Here's the drawing with two shaded views (mm, measured from the low corner). I have some questions. Coordinates: 2 decimals unless noted, no trailing zeros. Order: outer loops, then holes, each group sorted by start corner. A loop starts at its lowest first (then second) coordinate and runs counter-clockwise, first axis right, second up. Notation, with made-up numbers: (85, 74.5) - (93, 74.5) arc R17 cw to (93, 99.5) - close; hole circle Ø6 at (-14.75, 36). An arc over 180 degrees is marked (long way). Answer as a JSON object with one key per item and string values. Group by question number.
(1) Imagine slicing it at B-B, the plane x = 6.75. Write out the boundary of the cut face in (y, z) (1 decimal).
(2) We'd pull the mould along X, two halves only. Please class the marked faces 1, 2 and 3: pulls with the +X half, pulls with the -X half, needs draft (parallel to the pull), parting line crosses it, or undercut.
(3) Will this pin go through, and if not, where does the flat tip stop? P1, Ø1, axis at x = 3, z = 2, coming from the +Y side.
(4) Imagine slicing it at C-C, the plane z = 1.7. Write out the boundary of the cut face in (x, y) (1 decimal), and give its area (3 significant figures).
(5) Please list where these lines run through material, in increasing order: probe 1 along X at (y, z) = (8, 2.3) (1 decimal); probe 2 along Y at (x, z) = (6.5, 1.6) (1 decimal); probe 3 along Y at (x, z) = (5.75, 1.15) (1 decimal).
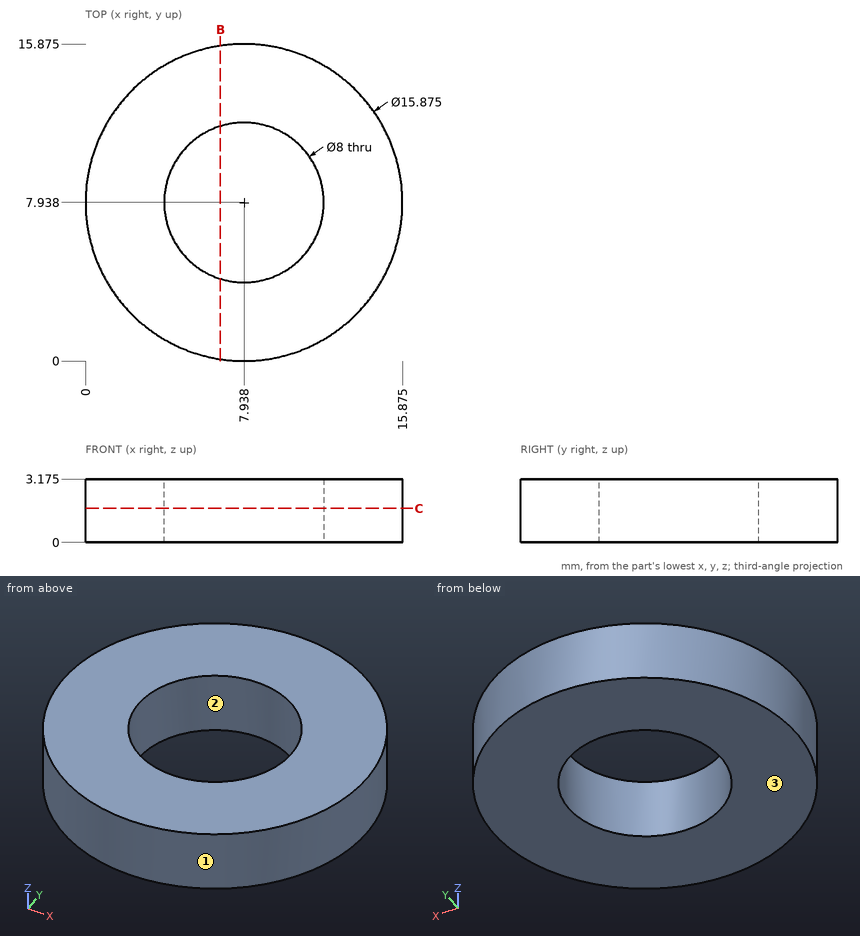
Result set:
{
 "1": {"outline": "(0.1, 0) - (4.1, 0) - (4.1, 3.2) - (0.1, 3.2) - close; (11.8, 0) - (15.8, 0) - (15.8, 3.2) - (11.8, 3.2) - close"},
 "2": {"face 1": "parting line crosses it", "face 2": "undercut", "face 3": "needs draft"},
 "3": {"P1": "stops at y = 14.52"},
 "4": {"outline": "circle Ø15.9 at (7.9, 7.9); hole circle Ø8 at (7.9, 7.9)", "area": "148 mm^2"},
 "5": {"probe 1": "x = 0 to 3.9, 11.9 to 15.9", "probe 2": "y = 0.1 to 4.2, 11.7 to 15.7", "probe 3": "y = 0.3 to 4.6, 11.3 to 15.6"}
}
